Here's how the part is built. I have some questions about the finished solid (model axes, mm). A direction names the side the tool comes from. Round coordinates to 2 decimals unless told otherwise and drop trailing zeros. Write each loop counter-clockwise with the first axis right and the second up, starting at its lowest first coordinate (ties: lowest second). Pieces come first, ordered by that corner, then holes. Notation, with made-up numbers: M -9.5,-16.75 L 21.5,-16.75 A15 cw 21.5,0.25 Z; hole C -24.5,-24 d8. An arc over 180 degrees is marked long. Write item = value, one per line. Start each with the question number.
(1) I want a section at C-C (z = 0). List the corners of the cut face in (x, y) for me, and give its area (3 significant figures).
(2) On a 3-axis mill with a long thin cutter (end or side, diameter ignored), from which of +Z, -Z, +X, -X, +Y, -Y can I reach the whole of each face in a straight line? I mean faces 1 (the flat face through (16.194, 9, 0)), 2 (the flat face through (18, 9, 5.113)), 3 (the flat face through (18, 9, -5.113)). Say none if no direction works.
(3) I need wall thicknesses on line 1 along Y through (x, z) = (4.5, -2.25); line 2 along X through (y, z) = (7.75, 4.5); line 3 along X through (y, z) = (0.75, -9). Which ranges of each line are inside material? Lowest first, please.
(4) Will these pins go through, and if not, where does the flat tip stop? pin 1 Ø3 at (y, z) = (8, -0.5) entering from -X; pin 2 Ø0.6 at (x, z) = (18.5, 0.5) entering from -Y; pin 3 Ø1 at (x, y) = (17.5, 7.5) entering from +Z.
(5) I want a section at D-D (x = 12). List the corners of the cut face in (y, z) for me, and give its area (3 significant figures).
(6) I want a section at B-B (x = 17). List the corners of the cut face in (y, z) for me, and give its area (3 significant figures).
(7) I want a section at A-A (z = -4.25). List the corners of the cut face in (x, y) for me.
```python
from build123d import *

# Parameters (mm, degrees)
SKETCH1_W           = 35
SKETCH1_H           = 20
BOSS_EXTRUDE1_DEPTH = 4
SKETCH2_W           = 3.466821798
SKETCH2_H           = 10.225967746
BOSS_EXTRUDE2_DEPTH = 10
SKETCH3_R           = 2.80007344
BOSS_EXTRUDE3_DEPTH = 1
BOSS_EXTRUDE3_TAPER = 30


with BuildPart() as part:
    # Sketch1 → Boss-Extrude1 (new body)
    with BuildSketch(Plane(origin=(0, 0, 0), x_dir=(1, 0, 0), z_dir=(0, 1, 0))):
        Rectangle(SKETCH1_W, SKETCH1_H)
    extrude(amount=BOSS_EXTRUDE1_DEPTH)

    # Sketch2 → Boss-Extrude2 (add)
    with BuildSketch(Plane(origin=(0, 4, 0), x_dir=(1, 0, 0), z_dir=(0, 1, 0))):
        with Locations((17.927516635, 0)):
            Rectangle(SKETCH2_W, SKETCH2_H)
    extrude(amount=BOSS_EXTRUDE2_DEPTH)

    # Sketch3 → Boss-Extrude3 (add)
    with BuildSketch(Plane(origin=(19.660927534, 0, 0), x_dir=(0, 0, -1), z_dir=(1, 0, 0))):
        with Locations((0, 10.617493758)):
            Circle(SKETCH3_R)
    extrude(amount=BOSS_EXTRUDE3_DEPTH, taper=BOSS_EXTRUDE3_TAPER)


solid = part.part
```
Returned:
q1.outline = M -17.5,0 L 17.5,0 L 17.5,4 L 19.66,4 L 19.66,7.82 L 20.66,8.39 L 20.66,12.84 L 19.66,13.42 L 19.66,14 L 16.19,14 L 16.19,4 L -17.5,4 Z
q1.area = 180 mm²
q2.face_1 = +Z, -Z, -X, +Y
q2.face_2 = +Z, +X, -X, +Y
q2.face_3 = -Z, +X, -X, +Y
q3.line_1 = 0 to 4
q3.line_2 = 16.19 to 19.66
q3.line_3 = -17.5 to 17.5
q4.pin_1 = 16.19
q4.pin_2 = 4
q4.pin_3 = 5.11
q5.outline = M 0,-10 L 4,-10 L 4,10 L 0,10 Z
q5.area = 80.0 mm²
q6.outline = M 0,-10 L 4,-10 L 4,-5.11 L 14,-5.11 L 14,5.11 L 4,5.11 L 4,10 L 0,10 Z
q6.area = 182 mm²
q7.outline = M -17.5,0 L 17.5,0 L 17.5,4 L 19.66,4 L 19.66,14 L 16.19,14 L 16.19,4 L -17.5,4 Z
